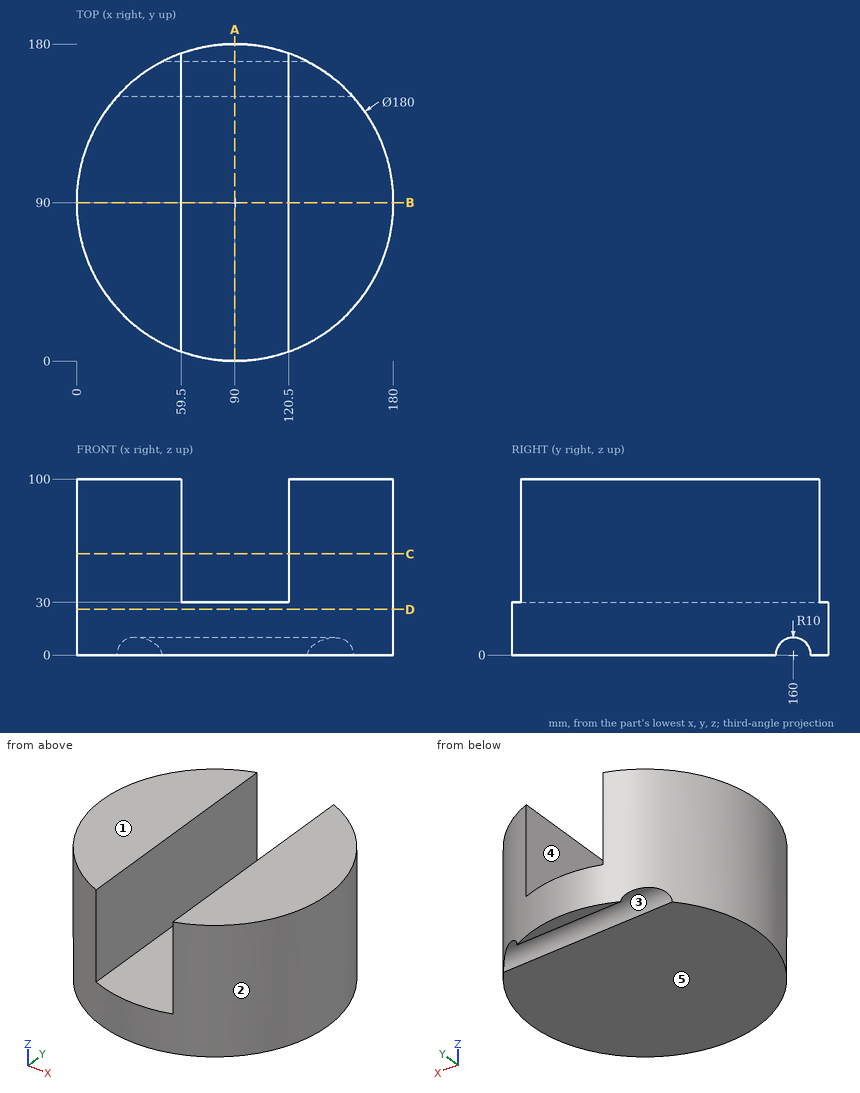
Answer from the drawing. Dimensions are ordinates in mm from the lowest x, y and z of the part. A direction names the side the tool comes from. Give positions to 0.01 mm unless a question says otherwise; leave off trailing zeros. Order: outer loops, then holes, each group sorted by start corner. A loop starts at its lowest first (then second) coordinate and runs counter-clockwise, first axis right, second up. Notation, with made-up numbers: (11, 58) - (61, 58) arc R35 cw to (61, 92) - close; hole circle Ø1 at (-33, 57). An arc over 180 degrees is marked (long way). One line per item, written item: value. Start each with the question number.
1. Section D-D, the plane z = 26 is taken. Write down the section's boundary in (x, y), then the cut area to 3 significant figures.
2. Section C-C, the plane z = 57.5 is taken. Write down the section's boundary in (x, y).
3. For a pull along Y with two mould halves and no side action, classify the marked faces 1, 2 and 3 as released by +Y, released by -Y, zero draft, split by the parting line, or undercut.
4. Section A-A, the plane x = 90 is taken. Write down the section's boundary in (y, z).
5. Consider line 1 (X direction, y = 30, z = 57.5); line 2 (Z direction, x = 118, y = 98.5); line 3 (X direction, y = 170.5, z = 35). Determine where each line is inside the solid, lowest interval first.
6. Which of the six approach directions +Z, -Z, +X, -X, +Y, -Y give full straight-line access (tool end or side, diameter ignored) to the marked faces 4 and 5?
7. Section B-B, the plane y = 90 is taken. Write down the section's boundary in (x, z), then the cut area to 3 significant figures.
8. Each of these flat-tipped pins is pushed along its axis until it touches: pin 1 Ø1.5 at (y, z) = (38, 52) entering from -X; pin 2 Ø12 at (x, y) = (72.5, 147) entering from +Z; pin 3 Ø4 at (x, z) = (57, 64.5) entering from +Y. Where does it stop, or does it pass through?
Filled sheet:
1. outline: circle Ø180 at (90, 90)
1. area: 25,400 mm²
2. outline: (59.5, 5.33) - (59.5, 174.67) arc R90 ccw to start; (120.5, 5.33) arc R90 ccw to (120.5, 174.67) - close
3. face 1: zero draft
3. face 2: split by the parting line
3. face 3: undercut
4. outline: (0, 0) - (150, 0) arc R10 cw to (170, 0) - (180, 0) - (180, 30) - (0, 30) - close
5. line 1: 22.92 to 59.5, 120.5 to 157.08
5. line 2: 0 to 30
5. line 3: 49.75 to 59.5, 120.5 to 130.25
6. face 4: +Z, +Y, -Y
6. face 5: -Z, +X, -X, +Y, -Y
7. outline: (0, 0) - (180, 0) - (180, 100) - (120.5, 100) - (120.5, 30) - (59.5, 30) - (59.5, 100) - (0, 100) - close
7. area: 13,700 mm²
8. pin 1: x = 16.02
8. pin 2: z = 30
8. pin 3: y = 174.49
